Geometry check sheet. Reference: the model listing, model coordinates, mm. Coordinates: 2 decimals unless noted, no trailing zeros. Loops run counter-clockwise (first coordinate to the right, second up) from the corner with the lowest first, then second, coordinate; pieces in that order, holes last. Notation, with made-up numbers: (65.25, 51) - (109.25, 51) arc R18 ccw to (109.25, 86) - close; hole circle Ø3 at (63.5, 4.5). An arc over 180 degrees is marked (long way). Write each question's results on one line, items separated by ' | '. Start each with the question number.
(1) Sectioned sample at A-A (y = 21.5). Enter the section's corners in (x, z), plus the area to 3 significant figures.
(2) Material ranges on probe 1 along X at (y, z) = (2.5, 2.6); probe 2 along X at (y, z) = (6.5, 0.45); probe 3 along X at (y, z) = (36, 2.8), recorded low to high.
(3) Sectioned sample at B-B (x = 65.5). Enter the section's corners in (y, z).
from build123d import *

# Parameters (mm, degrees)
BOSS_EXTRUDE1_DEPTH = 3
BOSS_EXTRUDE2_DEPTH = 3
SKETCH5_R           = 1.5
CUT_EXTRUDE7_DEPTH  = 7
SKETCH5_26_R        = 1.5
CUT_EXTRUDE8_DEPTH  = 7


with BuildPart() as part:
    # Sketch1 → Boss-Extrude1 (new body)
    with BuildSketch(Plane.XY):
        Polygon((-7, 40.912310071), (-7, 30.912310071), (-7, 4.912310071), (-7, -5.087689929), (5, -5.087689929), (69.955466391, -5.087689929), (84, -5.087689929), (84, 4.912310071), (84, 30.912310071), (84, 40.912310071), (69.955466391, 40.912310071), (5, 40.912310071), align=None)
        Polygon((20.466599793, 11.912310071), (21.466599793, 11.912310071), (21.466599793, 7.412310071), (26.966599793, 7.412310071), (26.966599793, 6.412310071), (21.466599793, 6.412310071), (21.466599793, 1.912310071), (20.466599793, 1.912310071), (20.466599793, 6.412310071), (14.966599793, 6.412310071), (14.966599793, 7.412310071), (20.466599793, 7.412310071), align=None, mode=Mode.SUBTRACT)
        Polygon((53.488866598, 7.412310071), (53.488866598, 11.912310071), (54.488866598, 11.912310071), (54.488866598, 7.412310071), (59.988866598, 7.412310071), (59.988866598, 6.412310071), (54.488866598, 6.412310071), (54.488866598, 1.912310071), (53.488866598, 1.912310071), (53.488866598, 6.412310071), (47.988866598, 6.412310071), (47.988866598, 7.412310071), align=None, mode=Mode.SUBTRACT)
        Polygon((40.5, 37.912310071), (40.5, 19.912310071), (67.477733195, 19.912310071), (67.477733195, 15.912310071), (40.5, 15.912310071), (40.5, -2.087689929), (36.5, -2.087689929), (36.5, 15.912310071), (7.477733195, 15.912310071), (7.477733195, 19.912310071), (36.5, 19.912310071), (36.5, 37.912310071), align=None, mode=Mode.SUBTRACT)
        Polygon((21.466599793, 28.412310071), (21.466599793, 23.912310071), (20.466599793, 23.912310071), (20.466599793, 28.412310071), (14.966599793, 28.412310071), (14.966599793, 29.412310071), (20.466599793, 29.412310071), (20.466599793, 33.912310071), (21.466599793, 33.912310071), (21.466599793, 29.412310071), (26.966599793, 29.412310071), (26.966599793, 28.412310071), align=None, mode=Mode.SUBTRACT)
        Polygon((54.488866598, 23.912310071), (53.488866598, 23.912310071), (53.488866598, 28.412310071), (47.988866598, 28.412310071), (47.988866598, 29.412310071), (53.488866598, 29.412310071), (53.488866598, 33.912310071), (54.488866598, 33.912310071), (54.488866598, 29.412310071), (59.988866598, 29.412310071), (59.988866598, 28.412310071), (54.488866598, 28.412310071), align=None, mode=Mode.SUBTRACT)
    extrude(amount=BOSS_EXTRUDE1_DEPTH)

    # Sketch3 → Boss-Extrude2 (add)
    with BuildSketch(Plane.XY.offset(3)):
        Polygon((-7, -5.087689929), (-7, 0.912310071), (0, 0.912310071), (0, -0.087689929), (5, -0.087689929), (5, -5.087689929), align=None)
        Polygon((0, 35.912310071), (5, 35.912310071), (5, 40.912310071), (-7, 40.912310071), (-7, 34.912310071), (0, 34.912310071), align=None)
        Polygon((77, -0.087689929), (72, -0.087689929), (72, -5.087689929), (84, -5.087689929), (84, 0.912310071), (77, 0.912310071), align=None)
        Polygon((77, 34.912310071), (77, 35.912310071), (72, 35.912310071), (72, 40.912310071), (84, 40.912310071), (84, 34.912310071), align=None)
    extrude(amount=BOSS_EXTRUDE2_DEPTH)

    # Sketch5 → Cut-Extrude7 (cut, through all)
    with BuildSketch(Plane.XY):
        with Locations((79.617691454, -1.9)):
            Circle(SKETCH5_R)
    extrude(amount=CUT_EXTRUDE7_DEPTH, mode=Mode.SUBTRACT)

    # Sketch5<26> → Cut-Extrude8 (cut, through all)
    with BuildSketch(Plane.XY):
        with Locations((-2.617691454, 37.9)):
            Circle(SKETCH5_26_R)
        with Locations((-2.617691454, -1.9)):
            Circle(SKETCH5_26_R)
        with Locations((79.617691454, 37.9)):
            Circle(SKETCH5_26_R)
    extrude(amount=CUT_EXTRUDE8_DEPTH, mode=Mode.SUBTRACT)


solid = part.part
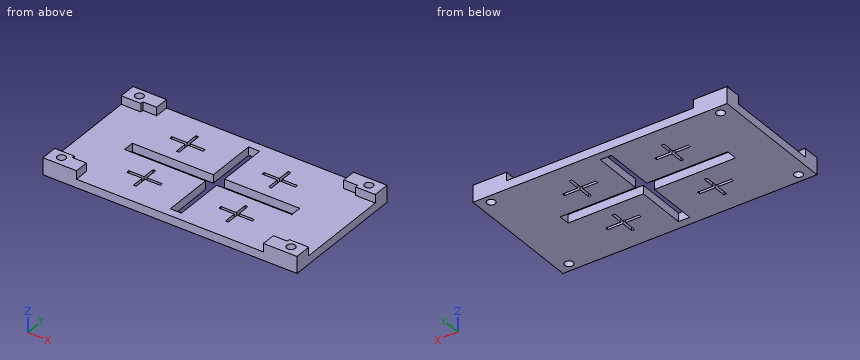
Outcome:
1) outline: (-7, 0) - (36.5, 0) - (36.5, 3) - (-7, 3) - close; (40.5, 0) - (84, 0) - (84, 3) - (40.5, 3) - close | area: 261 mm2
2) probe 1: x = -7 to 20.47, 21.47 to 36.5, 40.5 to 53.49, 54.49 to 84 | probe 2: x = -7 to 14.97, 26.97 to 36.5, 40.5 to 47.99, 59.99 to 84 | probe 3: x = -7 to 36.5, 40.5 to 84
3) outline: (-5.09, 0) - (15.91, 0) - (15.91, 3) - (-5.09, 3) - close; (19.91, 0) - (40.91, 0) - (40.91, 3) - (19.91, 3) - close
